```python
from build123d import *

# Parameters (mm, degrees)
CUT_EXTRUDE_1_DEPTH = 1.04
FILLET_1_R          = 0.1


with BuildPart() as part:
    # 草图1 → 旋转1 (revolve)
    with BuildSketch(Plane.XY):
        with BuildLine():
            Line((0, 2.304545455), (-1.8, 2.304545455))
            ThreePointArc((-1.8, 2.304545455), (-2.467032631, 1.569929856), (-2.85, 0.654545455))
            Line((-2.85, 0.654545455), (-1.5, 0.654545455))
            Line((-1.5, 0.654545455), (-1.5, -5.345454545))
            Line((-1.5, -5.345454545), (0, -5.345454545))
            Line((0, -5.345454545), (0, 2.304545455))
        make_face()
    revolve(axis=Axis((0, 0, 0), (0, 1, 0)))

    # 草图2 → 切除-拉伸1 (cut)
    with BuildSketch(Plane(origin=(0, 2.304545455, 0), x_dir=(1, 0, 0), z_dir=(0, 1, 0))):
        Polygon((0, -1.172021046), (1.015, -0.586010523), (1.015, 0.586010523), (0, 1.172021046), (-1.015, 0.586010523), (-1.015, -0.586010523), align=None)
    extrude(amount=-CUT_EXTRUDE_1_DEPTH, mode=Mode.SUBTRACT)

    # 圆角1
    fillet_1_edges = [part.edges().sort_by_distance(p)[0] for p in [
        (1.5, 0.654545455, 0),
    ]]
    fillet(fillet_1_edges, radius=FILLET_1_R)


solid = part.part
```
Build history of the part. All positions in model axes, mm. A direction names the side the tool comes from. Give positions to 0.01 mm unless a question says otherwise; leave off trailing zeros. Loops run counter-clockwise (first coordinate to the right, second up) from the corner with the lowest first, then second, coordinate; pieces in that order, holes last.
Item 1: Which spindle directions (+Z, -Z, +X, -X, +Y, -Y) get a long thin tool onto all of the face, cutting with end or side? Do faces 4 (the face through (0.515, 1.792, -0.875)), 5 (the face through (0, -5.345, 0)). Say none if no direction does.
Answers follow:
face 4: +Y
face 5: +Z, -Z, +X, -X, -Y
Item 2: Drill centre lines: line 1 (Y direction, x = -0.7, z = -1.55); line 2 (Y direction, x = 0.15, z = 1.05); line 3 (X direction, y = 0.75, z = 2.25). Where is each one in solid material? Low to high.
Answers follow:
line 1: y = 0.65 to 2.3
line 2: y = -5.35 to 1.26
line 3: x = -1.71 to 1.71
Item 3: Flat gauge pins, fed straight in: pin 1 (0.5 mm diameter, centred on y = 2, z = 0, fed in from -X); pin 2 (1 mm diameter, centred on y = -1.5, z = -0.5, fed in from -X); pin 3 (1.5 mm diameter, centred on x = 1.5, z = -2, fed in from -Y). Where does each tip first touch, or does it go through?
Answers follow:
pin 1: stops at x = -2.34
pin 2: stops at x = -1.5
pin 3: stops at y = 0.65
Item 4: Slice it at C-C, the plane z = -2.3. List the corners of the cut face in (x, y), and give its area (3 significant figures).
Answers follow:
outline: (-1.68, 0.65) - (1.68, 0.65) arc R1.81 ccw to start
area: 2.81 mm2
Item 5: Slice it at A-A, the plane z = 0. List the corners of the cut face in (x, y) (3 decimals), and give its area (3 significant figures).
Answers follow:
outline: (-2.85, 0.655) - (-1.6, 0.655) arc R0.1 cw to (-1.5, 0.555) - (-1.5, -5.345) - (1.5, -5.345) - (1.5, 0.555) arc R0.1 cw to (1.6, 0.655) - (2.85, 0.655) arc R2.924 ccw to (1.8, 2.305) - (1.015, 2.305) - (1.015, 1.265) - (-1.015, 1.265) - (-1.015, 2.305) - (-1.8, 2.305) arc R2.924 ccw to start
area: 24.0 mm2
Item 6: Slice it at B-B, the plane x = -2.35. List the corners of the cut face in (y, z).
Answers follow:
outline: (0.65, -1.61) arc R1.74 ccw to (0.65, 1.61) - close
Item 7: Pull direction Z, two halves, no side cores. Call faces 1 (the face through (1.015, 2, 0)), 2 (the face through (1.5, -2.44, 0.07)), 3 (the face through (0, 0.655, -2)): released by +Z, released by -Z, zero draft, split by the parting line, or undercut.
Answers follow:
face 1: undercut
face 2: split by the parting line
face 3: zero draft
